Input: part model. Units: mm. Frame: model coordinates. Coordinates: 2 decimals unless noted, no trailing zeros. Write each loop counter-clockwise with the first axis right and the second up, starting at its lowest first coordinate (ties: lowest second). Pieces come first, ordered by that corner, then holes. Notation, with made-up numbers: (-32, 40) - (2, 40) arc R21 cw to (2, 77) - close; hole circle Ø5 at (61, 41.5). An arc over 180 degrees is marked (long way). One line per question, with ' | ' between items. Start each with the question number.
1) Section query A-A on z = -10.75. Return loops of the section in (x, y) (3 decimals).
2) Line query: line 1 (X direction, y = -0.75, z = -12.25) (3 decimals); line 2 (Y direction, x = -0.75, z = -5); line 3 (Y direction, x = 0, z = -14.5). Output: solid intervals per line, ascending.
3) Draft query along Y for faces 1 (the conical face through (8.547, 4.962, -14.245)), 2 (the cylindrical face through (-0.749, 5.705, -7.36)), 3 (the conical face through (8.57, -4.92, -0.31)). Return one class per face: released by +Y, released by -Y, zero draft, split by the parting line, or undercut.
4) First-contact query: P1, Ø8, axis at x = -5.5, z = -10.5, coming from the +Y side; P2, Ø5, axis at x = 0, z = -7.5, coming from the -Y side; P3, Ø1.5, axis at y = -8.5, z = -3, coming from the -X side. Flat tips, straight axial feed; report the tip coordinate or a pass-through.
```python
from build123d import *

# Parameters (mm, degrees)
THREADSCHEMATIC_START     = -14.5542
THREADSCHEMATIC_OUTLINE_R = 5.75437
THREADSCHEMATIC_DEPTH     = 14.5542


# Read off the part's stored shape, not the designer's step: ThreadSchematic
with BuildPart() as part:
    # ThreadSchematic outline → ThreadSchematic (new body)
    with BuildSketch(Plane.XY.offset(THREADSCHEMATIC_START)):
        Polygon((9.525, 5.499261314), (0, 10.998522628), (-9.525, 5.499261314), (-9.525, -5.499261314), (0, -10.998522628), (9.525, -5.499261314), align=None)
        Circle(THREADSCHEMATIC_OUTLINE_R, mode=Mode.SUBTRACT)
    extrude(amount=THREADSCHEMATIC_DEPTH)

    # Sketch3 → Double-Chamfer (revolve, cut)
    with BuildSketch(Plane(origin=(0, 0, 0), x_dir=(0, 0, -1), z_dir=(1, 0, 0))):
        Polygon((14.5542, 9.525), (13.2842, 10.998522628), (13.2842, 23.698522628), (27.2542, 23.698522628), (27.2542, 9.525), align=None)
        Polygon((1.27, 23.698522628), (-12.7, 23.698522628), (-12.7, 9.525), (0, 9.525), (1.27, 10.998522628), align=None)
    revolve(axis=Axis((0, 0, 0), (0, 0, -1)), mode=Mode.SUBTRACT)

    # EndChamferSke → EndChamfer (revolve, cut)
    with BuildSketch(Plane(origin=(0, 0, 0), x_dir=(0, 0, -1), z_dir=(1, 0, 0)), mode=Mode.PRIVATE) as endchamfer_sk:
        Polygon((14.5288, 6.35), (14.070028922, 5.694807), (14.5796, 5.694807), (14.5796, 6.35), align=None)
        Polygon((-0.0508, 6.35), (0, 6.35), (0.458771078, 5.694807), (-0.0508, 5.694807), align=None)
    revolve(endchamfer_sk.sketch.rotate(Axis((0, 0, -25.037505729), (0, 0, -1)), 90), axis=Axis((0, 0, -25.037505729), (0, 0, -1)), mode=Mode.SUBTRACT)


solid = part.part
```
Answer key:
1) outline: (-9.525, -5.499) - (0, -10.999) - (9.525, -5.499) - (9.525, 5.499) - (0, 10.999) - (-9.525, 5.499) - close; hole circle Ø11.509 at (0, 0)
2) line 1: -9.525 to -5.705, 5.705 to 9.525 | line 2: -10.57 to -5.71, 5.71 to 10.57 | line 3: -9.59 to -6.31, 6.31 to 9.59
3) face 1: released by +Y | face 2: undercut | face 3: released by -Y
4) P1: y = 10.13 | P2: y = -11 | P3: x = -5.63
